Work out the finished part from the listing and answer in its coordinate system (mm). Round coordinates to 2 decimals unless told otherwise and drop trailing zeros. Write each loop counter-clockwise with the first axis right and the second up, starting at its lowest first coordinate (ties: lowest second). Pieces come first, ordered by that corner, then holes. Notation, with made-up numbers: M 13,-16.75 L 25,-16.75 A35 ccw 25,16.25 Z; hole C 49.5,-16.75 d3. An arc over 180 degrees is marked long. One line per item, written item: value. Start each with the question number.
Q1. Find section A-A (y = 38.04). Write down the section's boundary in (x, z).
Q2. Given pin 1 Ø4 at (y, z) = (188, 46) entering from -X; pin 2 Ø3 at (x, y) = (-459, 145.5) entering from -Z; pin 3 Ø0.8 at (x, y) = (-458, 161) entering from +Z, each flat-ended and moving along its own axis, determine where each tip first touches the part or whether it passes through.
Q3. Consider probe 1 along Y at (x, z) = (-458.45, 0); probe 2 along Y at (x, z) = (-458.85, 0); probe 3 along Z at (x, y) = (-459, 152). Determine where each line is inside the solid, lowest interval first.
Q4. Find section B-B (x = 0). Write down the section's boundary in (y, z), and give its area (3 significant figures).
Q5. Find section C-C (y = 232.5). Write down the section's boundary in (x, z), and give its area (3 significant figures).
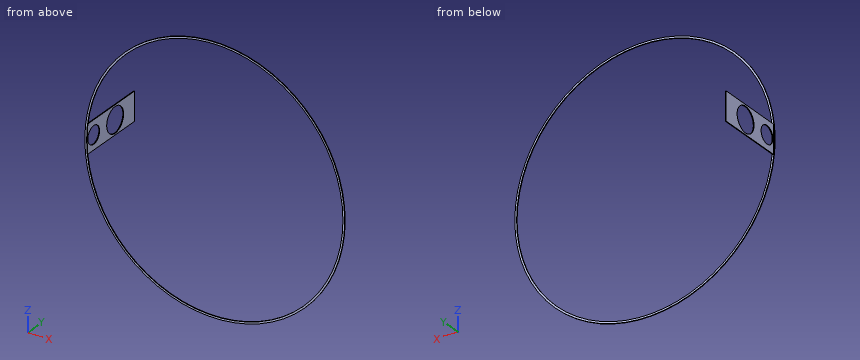
Autodesk Inventor part; units mm, degrees
ref_plane "YZ Plane" through (0, 0, 0) normal (1, 0, 0) x (0, 1, 0)
ref_plane "XZ Plane" through (0, 0, 0) normal (0, 1, 0) x (-1, 0, 0)
ref_plane "XY Plane" through (0, 0, 0) normal (0, 0, 1) x (1, 0, 0)
sketch "Sketch1" plane through (0, 0, 0) normal (0, 1, 0) x (-1, 0, 0)
  circle A0 centre (0, 0) radius 457.2
  circle A1 centre (0, 0) radius 463.55
  dimension "d0" = 914.4
  dimension "d1" = 6.35
extrude "Extrusion1" add sketch "Sketch1" along normal blind 2.54
sketch "Sketch2" plane through (0, 2.54, 0) normal (0, 1, 0) x (1, 0, 0)
  line L0 (-459.74, -50.8) -> (-457.2, -50.8)
  line L1 (-457.2, -50.8) -> (-457.2, 50.8)
  line L2 (-457.2, 50.8) -> (-459.74, 50.8)
  line L3 (-459.74, 50.8) -> (-459.74, -50.8)
  line L4 (-459.74, 0) -> (-457.2, 0) construction
  dimension "d4" = 2.54
  dimension "d5" = 101.6
extrude "Extrusion2" add sketch "Sketch2" along normal blind 254
sketch "Sketch3" plane through (0, 256.54, 0) normal (0, 1, 0) x (1, 0, 0)
  circle A0 centre (-458.47, 0) radius 0.254
  point P0 (0, 0)
  dimension "d8" = 0.508
extrude "Extrusion3" cut sketch "Sketch3" against normal blind 2.54
sketch "Sketch4" plane through (-459.74, 2.54, -50.8) normal (-1, 0, 0) x (0, 0, 1)
  line L0 (0, 254) -> (101.6, 254)
  circle A0 centre (50.8, 149.86) radius 45
  circle A1 centre (50.8, 35.5) radius 31.5
  point P0 (50.8, -2.54)
  dimension "d11" = 90
  dimension "d12" = 104.14
  dimension "d13" = 63
  dimension "d14" = 218.5
extrude "Extrusion4" cut sketch "Sketch4" against normal through all
equation "\"d0\" = hubOuterDiam"
equation "\"d11\" = sleeveOD"
equation "\"d13\" = sparOD"
equation "\"hubOuterDiam\" = 914.4"
equation "\"hubInnerDiam\" = 0.5 * hubOuterDiam"
equation "\"sleeveOD\" = 90"
equation "\"sparOD\" = 63"
properties part number "hubGuideRingOuter" material "Gold"
The answers:
1. outline: M -459.74,-50.8 L -457.2,-50.8 L -457.2,-31.5 L -459.74,-31.5 Z; M -459.74,31.5 L -457.2,31.5 L -457.2,50.8 L -459.74,50.8 Z
2. pin 1: x = -459.74
2. pin 2: z = -50.8
2. pin 3: z = 50.8
3. probe 1: 0 to 6.54, 69.54 to 107.4, 197.4 to 254
3. probe 2: 0 to 6.54, 69.54 to 107.4, 197.4 to 256.54
3. probe 3: -50.8 to -45, 45 to 50.8
4. outline: M 0,-463.55 L 2.54,-463.55 L 2.54,-457.2 L 0,-457.2 Z; M 0,457.2 L 2.54,457.2 L 2.54,463.55 L 0,463.55 Z
4. area: 32.3 mm2
5. outline: M -459.74,-50.8 L -457.2,-50.8 L -457.2,50.8 L -459.74,50.8 Z
5. area: 258 mm2
